```python
from build123d import *

# Parameters (mm, degrees)
SKETCH1_R                               = 57.15
BILLET_DEPTH                            = 10.16
KEROSENE_WELL_DEPTH                     = 6.35
FIRST_KEROSENE_OUTLET_REACH             = 83.458
SKETCH4_R                               = 0.7493
BOTTOM_NEEDLE_CHAMFER_SIZE              = 0.254
LPATTERN1_COUNT                         = 7
LPATTERN1_PITCH                         = 2.9972
LPATTERN1_COUNT_DIR2                    = 7
LPATTERN1_PITCH_DIR2                    = 2.9972
BOTTOM_NEEDLE_CHAMFER_OF_LPATTERN1_SIZE = 0.254
SKETCH13_R                              = 0.79375
DOWEL_HOLES_DEPTH                       = 3.175
MANIFOLD_HOLE_REACH                     = 83.458
SKETCH14_R                              = 3.175
SKETCH15_R                              = 56.515
SKETCH15_R_2                            = 54.61
CHAMBER_O_RING_DEPTH                    = 2.032
CUT_EXTRUDE4_START                      = -2.032
SKETCH16_R                              = 54.61
SKETCH16_R_2                            = 52.705
CUT_EXTRUDE4_DEPTH                      = 2.032


with BuildPart() as part:
    # Sketch1 → Billet (new body)
    with BuildSketch(Plane(origin=(0, 0, 0), x_dir=(1, 0, 0), z_dir=(0, 1, 0))):
        with Locations(Location((0, 0, 0), (0, 0, 270))):
            Circle(SKETCH1_R)
    extrude(amount=-BILLET_DEPTH)

    # Sketch2 → Kerosene Well (cut)
    with BuildSketch(Plane(origin=(0, 0, 0), x_dir=(1, 0, 0), z_dir=(0, 1, 0))):
        with BuildLine():
            Line((-31.75, 11.43), (31.75, 11.43))
            ThreePointArc((31.75, 11.43), (43.18, 0), (31.75, -11.43))
            Line((31.75, -11.43), (-31.75, -11.43))
            ThreePointArc((-31.75, -11.43), (-43.18, 0), (-31.75, 11.43))
        make_face()
    extrude(amount=-KEROSENE_WELL_DEPTH, mode=Mode.SUBTRACT)

    # Sketch4 → First Kerosene Outlet (cut, up to next)
    with BuildSketch(Plane(origin=(0, -10.16, 0), x_dir=(1, 0, 0), z_dir=(0, 1, 0)), mode=Mode.PRIVATE) as first_kerosene_outlet_sk1:
        with Locations(Location((8.9916, 8.9916, 0), (0, 0, 90))):
            Circle(SKETCH4_R)
    first_kerosene_outlet_tool1 = extrude(first_kerosene_outlet_sk1.sketch, amount=FIRST_KEROSENE_OUTLET_REACH, mode=Mode.PRIVATE) & part.part
    first_kerosene_outlet = first_kerosene_outlet_tool1.solids().sort_by_distance((8.9916, -10.16, -8.9916))[0]
    add(first_kerosene_outlet, mode=Mode.SUBTRACT)

    # Bottom Needle Chamfer
    bottom_needle_chamfer_edges = [part.edges().sort_by_distance(p)[0] for p in [
        (8.9916, -6.35, -8.2423),
    ]]
    chamfer(bottom_needle_chamfer_edges, length=BOTTOM_NEEDLE_CHAMFER_SIZE)

    # LPattern1: First Kerosene Outlet 7 × 7, 5 skipped
    with Locations(*[(-j * LPATTERN1_PITCH_DIR2, 0, i * LPATTERN1_PITCH) for i in range(LPATTERN1_COUNT) for j in range(LPATTERN1_COUNT_DIR2) if (i, j) not in ((0, 0), (2, 2), (2, 4), (3, 3), (4, 2), (4, 4))]):
        add(first_kerosene_outlet, mode=Mode.SUBTRACT)

    # Bottom Needle Chamfer of LPattern1
    bottom_needle_chamfer_of_lpattern1_edges = [part.edges().sort_by_distance(p)[0] for p in [
        (5.9944, -6.35, -8.2423),
        (2.9972, -6.35, -8.2423),
        (0, -6.35, -8.2423),
        (-2.9972, -6.35, -8.2423),
        (-5.9944, -6.35, -8.2423),
        (-8.9916, -6.35, -8.2423),
        (8.9916, -6.35, -5.2451),
        (5.9944, -6.35, -5.2451),
        (2.9972, -6.35, -5.2451),
        (0, -6.35, -5.2451),
        (-2.9972, -6.35, -5.2451),
        (-5.9944, -6.35, -5.2451),
        (-8.9916, -6.35, -5.2451),
        (8.9916, -6.35, -2.2479),
        (5.9944, -6.35, -2.2479),
        (0, -6.35, -2.2479),
        (-5.9944, -6.35, -2.2479),
        (-8.9916, -6.35, -2.2479),
        (8.9916, -6.35, 0.7493),
        (5.9944, -6.35, 0.7493),
        (2.9972, -6.35, 0.7493),
        (-2.9972, -6.35, 0.7493),
        (-5.9944, -6.35, 0.7493),
        (-8.9916, -6.35, 0.7493),
        (8.9916, -6.35, 3.7465),
        (5.9944, -6.35, 3.7465),
        (0, -6.35, 3.7465),
        (-5.9944, -6.35, 3.7465),
        (-8.9916, -6.35, 3.7465),
        (8.9916, -6.35, 6.7437),
        (5.9944, -6.35, 6.7437),
        (2.9972, -6.35, 6.7437),
        (0, -6.35, 6.7437),
        (-2.9972, -6.35, 6.7437),
        (-5.9944, -6.35, 6.7437),
        (-8.9916, -6.35, 6.7437),
        (8.9916, -6.35, 9.7409),
        (5.9944, -6.35, 9.7409),
        (2.9972, -6.35, 9.7409),
        (0, -6.35, 9.7409),
        (-2.9972, -6.35, 9.7409),
        (-5.9944, -6.35, 9.7409),
        (-8.9916, -6.35, 9.7409),
    ]]
    chamfer(bottom_needle_chamfer_of_lpattern1_edges, length=BOTTOM_NEEDLE_CHAMFER_OF_LPATTERN1_SIZE)

    # Sketch13 → Dowel Holes (cut)
    with BuildSketch(Plane(origin=(0, 0, 0), x_dir=(1, 0, 0), z_dir=(0, 1, 0))):
        with Locations(Location((0, 15.24, 0), (0, 0, 270))):
            Circle(SKETCH13_R)
        with Locations(Location((0, -15.24, 0), (0, 0, 90))):
            Circle(SKETCH13_R)
    extrude(amount=-DOWEL_HOLES_DEPTH, mode=Mode.SUBTRACT)

    # Sketch14 → Manifold Hole (cut, up to next)
    with BuildSketch(Plane(origin=(0, 0, 0), x_dir=(1, 0, 0), z_dir=(0, 1, 0)), mode=Mode.PRIVATE) as manifold_hole_sk1:
        with Locations(Location((0, 33.02, 0), (0, 0, 270))):
            Circle(SKETCH14_R)
    manifold_hole_tool1 = extrude(manifold_hole_sk1.sketch, amount=-MANIFOLD_HOLE_REACH, mode=Mode.PRIVATE) & part.part
    add(manifold_hole_tool1.solids().sort_by_distance((0, 0, -33.02))[0], mode=Mode.SUBTRACT)

    # Sketch15 → Chamber O Ring (cut)
    with BuildSketch(Plane(origin=(0, -10.16, 0), x_dir=(1, 0, 0), z_dir=(0, 1, 0))):
        with Locations(Location((0, 0, 0), (0, 0, 270))):
            Circle(SKETCH15_R)
        with Locations(Location((0, 0, 0), (0, 0, 270))):
            Circle(SKETCH15_R_2, mode=Mode.SUBTRACT)
    extrude(amount=CHAMBER_O_RING_DEPTH, mode=Mode.SUBTRACT)

    # Sketch16 → Cut-Extrude4 (cut)
    with BuildSketch(Plane(origin=(0, 0, 0), x_dir=(1, 0, 0), z_dir=(0, 1, 0)).offset(CUT_EXTRUDE4_START)):
        with Locations(Location((0, 0, 0), (0, 0, 270))):
            Circle(SKETCH16_R)
        with Locations(Location((0, 0, 0), (0, 0, 270))):
            Circle(SKETCH16_R_2, mode=Mode.SUBTRACT)
    extrude(amount=CUT_EXTRUDE4_DEPTH, mode=Mode.SUBTRACT)


solid = part.part
```
Here's how the part is built. I have some questions about the finished solid (model axes, mm). A direction names the side the tool comes from. Round coordinates to 2 decimals unless told otherwise and drop trailing zeros. Loops run counter-clockwise (first coordinate to the right, second up) from the corner with the lowest first, then second, coordinate; pieces in that order, holes last.
1. Suppose I cut it at C-C, the plane z = 13. Please give me the cut outline in (x, y).
Answers:
outline: (-55.65, -10.16) - (-55, -10.16) - (-55, -8.13) - (-53.04, -8.13) - (-53.04, -10.16) - (53.04, -10.16) - (53.04, -8.13) - (55, -8.13) - (55, -10.16) - (55.65, -10.16) - (55.65, 0) - (53.04, 0) - (53.04, -2.03) - (51.08, -2.03) - (51.08, 0) - (-51.08, 0) - (-51.08, -2.03) - (-53.04, -2.03) - (-53.04, 0) - (-55.65, 0) - close
2. Suppose I cut it at B-B, the plane x = 48. Please give me the cut outline in (y, z), and give its area (3 significant figures).
Answers:
outline: (-10.16, -31.02) - (0, -31.02) - (0, -26.04) - (-2.03, -26.04) - (-2.03, -21.77) - (0, -21.77) - (0, 21.77) - (-2.03, 21.77) - (-2.03, 26.04) - (0, 26.04) - (0, 31.02) - (-10.16, 31.02) - (-10.16, 29.83) - (-8.13, 29.83) - (-8.13, 26.04) - (-10.16, 26.04) - (-10.16, -26.04) - (-8.13, -26.04) - (-8.13, -29.83) - (-10.16, -29.83) - close
area: 598 mm2
3. Suppose I cut it at D-D, the plane x = 35. Please give me the cut outline in (y, z), and give its area (3 significant figures).
Answers:
outline: (-10.16, -45.18) - (0, -45.18) - (0, -41.92) - (-2.03, -41.92) - (-2.03, -39.41) - (0, -39.41) - (0, -10.96) - (-6.35, -10.96) - (-6.35, 10.96) - (0, 10.96) - (0, 39.41) - (-2.03, 39.41) - (-2.03, 41.92) - (0, 41.92) - (0, 45.18) - (-10.16, 45.18) - (-10.16, 44.37) - (-8.13, 44.37) - (-8.13, 41.92) - (-10.16, 41.92) - (-10.16, -41.92) - (-8.13, -41.92) - (-8.13, -44.37) - (-10.16, -44.37) - close
area: 759 mm2
4. Suppose I cut it at A-A, the plane z = -32. Please give me the cut outline in (x, y), and give its area (3 significant figures).
Answers:
outline: (-47.35, -10.16) - (-46.58, -10.16) - (-46.58, -8.13) - (-44.25, -8.13) - (-44.25, -10.16) - (-3.01, -10.16) - (-3.01, 0) - (-41.88, 0) - (-41.88, -2.03) - (-44.25, -2.03) - (-44.25, 0) - (-47.35, 0) - close; (3.01, -10.16) - (44.25, -10.16) - (44.25, -8.13) - (46.58, -8.13) - (46.58, -10.16) - (47.35, -10.16) - (47.35, 0) - (44.25, 0) - (44.25, -2.03) - (41.88, -2.03) - (41.88, 0) - (3.01, 0) - close
area: 882 mm2
5. For faces 5 (the face through (55.3, -10.16, -13)), 6 (the face through (1, -6.35, 0)), 7 (the face through (30, -8.128, -46)), which set-ups out of +Z, -Z, +X, -X, +Y, -Y let a thin tool reach every point of the face, with its end or its side?
Answers:
face 5: +Z, -Z, +X, -X, -Y
face 6: +Y
face 7: -Y
6. If I drill on probe 1 along Z at (x, y) = (-31, -1); probe 2 along Z at (x, y) = (-39, -8.5); probe 3 along Z at (x, y) = (30, -2), over which ranges is the centre line in solid material (lowest first)?
Answers:
probe 1: z = -48.01 to -44.96, -42.62 to -11.43, 11.43 to 42.62, 44.96 to 48.01
probe 2: z = -41.77 to -40.9, -38.23 to 38.23, 40.9 to 41.77
probe 3: z = -48.64 to -45.63, -43.33 to -11.43, 11.43 to 43.33, 45.63 to 48.64
7. Thinking about a two-plate mould opening in X: for faces 1 (the face through (46.047, -1.03, 29.358)), 2 (the face through (-43.177, -3.131, 0.251)), 3 (the face through (-29.4, 0, 46.3)), 4 (the face through (2.513, -5.009, -57.095)), which applies, released by +X, released by -X, zero draft, split by the parting line, or undercut?
Answers:
face 1: undercut
face 2: undercut
face 3: zero draft
face 4: split by the parting line
8. Will these pins go through, and if not, where does the flat tip stop? pin 1 (1.5 mm diameter, centred on y = -2, z = 40, fed in from +X); pin 2 (1.3 mm diameter, centred on x = 0, z = -3, fed in from -Y); pin 3 (5 mm diameter, centred on x = -3.5, z = 19, fed in from +Y); pin 4 (1.7 mm diameter, centred on x = 5.99, z = -3, fed in from +Y).
Answers:
pin 1: stops at x = 41.54
pin 2: passes through
pin 3: stops at y = 0
pin 4: stops at y = -6.5
